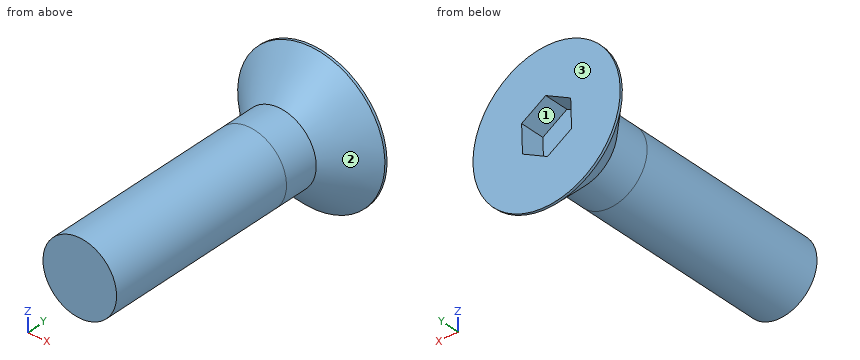
```python
from build123d import *

# Parameters (mm, degrees)
SKETCH_1_R          = 1.5
EXTRUDE_1_DEPTH     = 8
SKETCH_2_R          = 3
EXTRUDE_2_DEPTH     = 3
CHAMFER_1_SIZE      = 2.9
CUT_EXTRUDE_1_DEPTH = 1


with BuildPart() as part:
    # 草图1 → 凸台-拉伸1 (new body)
    with BuildSketch(Plane(origin=(0, 0, 0), x_dir=(1, 0, 0), z_dir=(0, 1, 0))):
        with Locations(Location((0, 0, 0), (0, 0, 270))):
            Circle(SKETCH_1_R)
    extrude(amount=EXTRUDE_1_DEPTH)

    # 草图2 → 凸台-拉伸2 (add)
    with BuildSketch(Plane(origin=(0, 8, 0), x_dir=(1, 0, 0), z_dir=(0, 1, 0))):
        with Locations(Location((0, 0, 0), (0, 0, 270))):
            Circle(SKETCH_2_R)
    extrude(amount=EXTRUDE_2_DEPTH)

    # 倒角1
    # the kernel refuses this chamfer: 2.9 mm, written as the material it takes off along each edge
    with BuildSketch(Plane(origin=(0, 8, 0), x_dir=(0, 0, 1), z_dir=(-1, 0, 0))) as chamfer_1_piece_1_section:
        Polygon((3, CHAMFER_1_SIZE), (3 - CHAMFER_1_SIZE, 0), (3, 0), align=None)
    chamfer_1_piece_1 = revolve(axis=Axis((0, 8, 0), (0, 1, 0)), mode=Mode.PRIVATE)
    chamfer_1_piece_1 = chamfer_1_piece_1 - Plane(origin=(0, 10.16453564, 0), x_dir=(0, 0, 1), z_dir=(0, -1, 0)) * Cylinder(1.5, 12, mode=Mode.PRIVATE)
    add(chamfer_1_piece_1, mode=Mode.SUBTRACT)

    # 草图3 → 切除-拉伸1 (cut)
    with BuildSketch(Plane(origin=(0, 11, 0), x_dir=(1, 0, 0), z_dir=(0, 1, 0))):
        Polygon((1.017530084, -0.545862493), (0.981495828, 0.608275655), (-0.036034256, 1.154138148), (-1.017530084, 0.545862493), (-0.981495828, -0.608275655), (0.036034256, -1.154138148), align=None)
    extrude(amount=-CUT_EXTRUDE_1_DEPTH, mode=Mode.SUBTRACT)


solid = part.part
```
For this review, take the finished solid that the model builds, in its own axes (mm). Face numbers are marked on the shaded views. Give positions to 0.01 mm unless a question says otherwise; leave off trailing zeros. Write each loop counter-clockwise with the first axis right and the second up, starting at its lowest first coordinate (ties: lowest second). Pieces come first, ordered by that corner, then holes.
Item 1: Insertion check: P1, Ø2, axis at x = -0.5, z = -1, coming from the -Y side; P2, Ø1, axis at x = 0, z = 0, coming from the +Y side; P3, Ø3, axis at x = -2, y = 6, coming from the -Z side; P4, Ø2, axis at x = 2, y = 2, coming from the +Z side. Each pin has a flat end and moves straight along its axis. Give the tip position at first contact, or say it passes through.
Item 2: Take a section at B-B (y = 3.25). Give the boundary of the cut face in (x, z), and give its area (3 significant figures).
Item 3: Wall thickness on probe 1 along Y at (x, z) = (-0.9, 0.1); probe 2 along X at (y, z) = (4.5, 1.1); probe 3 along X at (y, z) = (7.5, -0.9): over which ranges is each line inside the solid? List them lowest first.
Item 4: Take a section at A-A (z = 0). Give the boundary of the cut face in (x, y).
Item 5: The part is to be moulded in two halves that separate along X. For the marked faces 1, 2 and 3, say which applies: +X half, -X half, draft (parallel to the pull), parting line (faces both ways), or undercut.
Established:
1. P1: stops at y = 0
1. P2: stops at y = 10
1. P3: stops at z = -1.41
1. P4: stops at z = 1.12
2. outline: circle Ø3 at (0, 0)
2. area: 7.07 mm2
3. probe 1: y = 0 to 10
3. probe 2: x = -1.02 to 1.02
3. probe 3: x = -1.2 to 1.2
4. outline: (-3, 10.9) - (-1.5, 9.4) - (-1.5, 0) - (1.5, 0) - (1.5, 9.4) - (3, 10.9) - (3, 11) - (1, 11) - (1, 10) - (-1, 10) - (-1, 11) - (-3, 11) - close
5. face 1: undercut
5. face 2: parting line
5. face 3: draft
